Work out the finished part from the listing and answer in its coordinate system (mm). A direction names the side the tool comes from. Coordinates: 2 decimals unless noted, no trailing zeros. Order: outer loops, then holes, each group sorted by start corner. A loop starts at its lowest first (then second) coordinate and runs counter-clockwise, first axis right, second up. Notation, with made-up numbers: (76, 72) -> (87, 72) arc R16 cw to (87, 93) -> close; hole circle Ø11 at (71.25, 7.25). An arc over 180 degrees is marked (long way). Write item = value, one per line. Start each with the question number.
Q1. Straight lines are drawn through the part: L1, parallel to Z at x = -21, y = -14.85; L2, parallel to Y at x = 18.5, z = 4.4; L3, parallel to Y at x = 0, z = 2.85. For each, find the intervals that lie inside material, in ascending order. Write a range as from..to.
Q2. The part is cut by section B-B, the plane z = 4. Determine the outline of the cut face in (x, y).
Q3. The part is cut by section A-A, the plane x = 21. Determine the outline of the cut face in (y, z).
Q4. For a pull along Y with two mould halves and no side action, classify faces 3 (the cylindrical face through (0, 16, 3)), 4 (the flat face through (-1.7, -12.3, 0)), 5 (the flat face through (0, -16, 3)) as +Y half, -Y half, draft (parallel to the pull), parting line (faces both ways), or undercut.
Q5. Which of the six approach directions +Z, -Z, +X, -X, +Y, -Y give full straight-line access (tool end or side, diameter ignored) to faces 1 (the cylindrical face through (13.214, -11.959, 3.042)), 2 (the cylindrical face through (-17.699, -16.285, 3.042))?
Q6. Flat-ended cylindrical pins translate along their axes: pin 1 (1.8 mm diameter, centred on x = -6.5, z = 3, fed in from -Y); pin 2 (2 mm diameter, centred on y = 5.5, z = 3.5, fed in from +X); pin 3 (3.5 mm diameter, centred on x = 21, z = 3, fed in from +Y). Find the tip coordinate at first contact, or state that the pin passes through.
Q7. The part is cut by section C-C, the plane y = 0. Determine the outline of the cut face in (x, z).
```python
from build123d import *

# Parameters (mm, degrees)
SKETCH1_R             = 12.2
BOSS_EXTRUDE1_DEPTH   = 6
FILLET1_R             = 3
FILLET2_R             = 1
F_3_0MM_DOWEL_HOLE1_D = 3.2


with BuildPart() as part:
    # Sketch1 → Boss-Extrude1 (new body)
    with BuildSketch(Plane.XY):
        with BuildLine():
            Line((18, -16), (-18, -16))
            Line((-18, -16), (-18, -18))
            Line((-18, -18), (-24, -18))
            Line((-24, -18), (-24, -13.5))
            Line((-24, -13.5), (-8.587782019, -13.5))
            ThreePointArc((-8.587782019, -13.5), (0, 16), (8.587782019, -13.5))
            Line((8.587782019, -13.5), (24, -13.5))
            Line((24, -13.5), (24, -18))
            Line((24, -18), (18, -18))
            Line((18, -18), (18, -16))
        make_face()
        Circle(SKETCH1_R, mode=Mode.SUBTRACT)
    extrude(amount=BOSS_EXTRUDE1_DEPTH)

    # Fillet1
    fillet1_edges = [part.edges().sort_by_distance(p)[0] for p in [
        (-8.587782019, -13.5, 3),
        (8.587782019, -13.5, 3),
    ]]
    fillet(fillet1_edges, radius=FILLET1_R)

    # Fillet2
    fillet2_edges = [part.edges().sort_by_distance(p)[0] for p in [
        (18, -16, 3),
        (-18, -16, 3),
    ]]
    fillet(fillet2_edges, radius=FILLET2_R)

    # Ø3.0mm Dowel Hole1 (through all)
    with Locations(Plane(origin=(0, -13.5, 0), x_dir=(1, 0, 0), z_dir=(0, 1, 0))):
        with Locations((-21, -3), (21, -3)):
            Hole(F_3_0MM_DOWEL_HOLE1_D / 2)


solid = part.part
```
Model answer:
q1.L1 = 0..1.4, 4.6..6
q1.L2 = -18..-13.5
q1.L3 = -16..-12.2, 12.2..16
q2.outline = (-24, -18) -> (-22.25, -18) -> (-22.25, -13.5) -> (-24, -13.5) -> close; (-19.75, -18) -> (-18, -18) -> (-18, -17) arc R1 cw to (-17, -16) -> (17, -16) arc R1 cw to (18, -17) -> (18, -18) -> (19.75, -18) -> (19.75, -13.5) -> (15.84, -13.5) arc R3 cw to (13.33, -8.84) arc R16 ccw (long way) to (-13.33, -8.84) arc R3 cw to (-15.84, -13.5) -> (-19.75, -13.5) -> close; (22.25, -18) -> (24, -18) -> (24, -13.5) -> (22.25, -13.5) -> close; hole circle Ø24.4 at (0, 0)
q3.outline = (-18, 0) -> (-13.5, 0) -> (-13.5, 1.4) -> (-18, 1.4) -> close; (-18, 4.6) -> (-13.5, 4.6) -> (-13.5, 6) -> (-18, 6) -> close
q4.face_3 = undercut
q4.face_4 = draft
q4.face_5 = -Y half
q5.face_1 = +Z, -Z, +X
q5.face_2 = +Z, -Z, -Y
q6.pin_1 = -16
q6.pin_2 = 15.35
q6.pin_3 = -13.5
q7.outline = (-16, 0) -> (-12.2, 0) -> (-12.2, 6) -> (-16, 6) -> close; (12.2, 0) -> (16, 0) -> (16, 6) -> (12.2, 6) -> close
